Here's how the part is built. I have some questions about the finished solid (model axes, mm). A direction names the side the tool comes from. Round coordinates to 2 decimals unless told otherwise and drop trailing zeros. Loops run counter-clockwise (first coordinate to the right, second up) from the corner with the lowest first, then second, coordinate; pieces in that order, holes last. Notation, with made-up numbers: M 69,-20 L 100,-20 A10 cw 100,-7 Z; hole C -28,28.25 d6. An arc over 180 degrees is marked long. Use a Markdown table: item, result.
```python
from build123d import *

# Parameters (mm, degrees)
F0_R      = 8.9296875
F0_R_2    = 3.96875
F0_R_3    = 3.175
F0_R_4    = 1.68671875
F1_DEPTH  = 3.175
F2_DEPTH  = 1.3208
F3_DEPTH  = 6.0833
F1_FACE_R = 8.9296875


# Not quite as in the source:
# - a length typed as a fraction of an inch, garbled in the dataset ("3 / 203.2 mm" for 3/8 in), is restored


with BuildPart() as f1:
    # F0 (on Top) → F1 (new body)
    with BuildSketch(Plane.XY):
        Circle(F0_R)
        Circle(F0_R_2, mode=Mode.SUBTRACT)
        Circle(F0_R_2)
        Circle(F0_R_3, mode=Mode.SUBTRACT)
        Circle(F0_R_3)
        Circle(F0_R_4, mode=Mode.SUBTRACT)
        Circle(F0_R_4)
    extrude(amount=-F1_DEPTH)

    # F0 (on Top) → F2 (join)
    with BuildSketch(Plane.XY):
        Circle(F0_R_2)
        Circle(F0_R_3, mode=Mode.SUBTRACT)
        Circle(F0_R_3)
        Circle(F0_R_4, mode=Mode.SUBTRACT)
        Circle(F0_R_4)
    extrude(amount=F2_DEPTH)

    # F0 (on Top) → F3 (join)
    with BuildSketch(Plane.XY):
        Circle(F0_R_4)
    extrude(amount=F3_DEPTH)

    # F1_face (on face) → F4 section 0
    with BuildSketch(Plane(origin=(0, 0, -3.175), x_dir=(1, 0, 0), z_dir=(0, 0, -1)), mode=Mode.PRIVATE) as f4_s0:
        Circle(F1_FACE_R)
    loft([f4_s0.sketch, Vertex(0, 0, 0)], mode=Mode.SUBTRACT)


solid = f1.part
```
Q1. Will these pins go through, and if not, where does the flat tip stop? P1, Ø4, axis at y = -5.5, z = 3.5, coming from the -X side; P2, Ø1.5, axis at x = 6.5, y = 4.5, coming from the +Z side; P3, Ø8, axis at x = 4, y = 6, coming from the +Z side; P4, Ø5, axis at x = 2.5, y = 3, coming from the -Z side.
Return value:
| item | result |
|---|---|
| P1 | passes through |
| P2 | stops at z = 0 |
| P3 | stops at z = 1.32 |
| P4 | stops at z = -2.28 |
Q2. I need wall thicknesses on line 1 (X direction, y = 1, z = 3.25); line 2 (Z direction, x = -5.25, y = -2.5); line 3 (Y direction, x = 1.5, z = 0.25). Which ranges of each line are inside material? Lowest first, please. Write a range as from..to.
Return value:
| item | result |
|---|---|
| line 1 | x = -1.36..1.36 |
| line 2 | z = -2.07..0 |
| line 3 | y = -3.67..3.67 |
Q3. For faces 1 (the cylindrical face through (-8.92, 0.39, -1.57)), 2 (the cylindrical face through (-1.243, 1.14, 3.669)), which set-ups out of +Z, -Z, +X, -X, +Y, -Y let a thin tool reach every point of the face, with its end or its side?
Return value:
| item | result |
|---|---|
| face 1 | +Z, -Z |
| face 2 | +Z |
Q4. Imagine slicing it at A-A, the plane z = 2.75. Please give me the cut outline in (x, y).
Return value:
| item | result |
|---|---|
| outline | C 0,0 d3.37 |
Q5. Imagine slicing it at B-B, the plane z = -1.25. Please give me the cut outline in (x, y), then the cut area to 3 significant figures.
Return value:
| item | result |
|---|---|
| outline | C 0,0 d17.86; hole C 0,0 d7.03 |
| area | 212 mm^2 |
Q6. Imagine slicing it at C-C, the plane z = 0.75. Please give me the cut outline in (x, y).
Return value:
| item | result |
|---|---|
| outline | C 0,0 d7.94 |
Q7. We'd pull the mould along X, two halves only. Please class faces 3 (the conical face through (0, 0, 0)), 4 (the cylindrical face through (-0.86, -3.874, 0.651)), 5 (the flat face through (2, -4, 0)): pulls with the +X half, pulls with the -X half, needs draft (parallel to the pull), parting line crosses it, or undercut.
Return value:
| item | result |
|---|---|
| face 3 | undercut |
| face 4 | parting line crosses it |
| face 5 | needs draft |
